```python
from build123d import *

# Parameters (mm, degrees)
SKETCH1_W           = 20.32
SKETCH1_H           = 42
BOSS_EXTRUDE1_DEPTH = 1.5748
SKETCH2_W           = 42
SKETCH2_H           = 1.5748
BOSS_EXTRUDE2_DEPTH = 62.32
SKETCH3_R           = 11.303
SKETCH3_R_2         = 1.6891
CUT_EXTRUDE1_DEPTH  = 62.32
SKETCH4_R           = 2.05
CUT_EXTRUDE2_DEPTH  = 62.32


with BuildPart() as part:
    # Sketch1 → Boss-Extrude1 (new body)
    with BuildSketch(Plane(origin=(0, 0, 0), x_dir=(0, 1, 0), z_dir=(0, 0, 1))):
        Rectangle(SKETCH1_W, SKETCH1_H)
    extrude(amount=BOSS_EXTRUDE1_DEPTH)

    # Sketch2 → Boss-Extrude2 (add)
    with BuildSketch(Plane.XY.offset(1.5748)):
        with Locations((0, 9.3726)):
            Rectangle(SKETCH2_W, SKETCH2_H)
    extrude(amount=BOSS_EXTRUDE2_DEPTH)

    # Sketch3 → Cut-Extrude1 (cut)
    with BuildSketch(Plane(origin=(0, 8.5852, 0), x_dir=(-1, 0, 0), z_dir=(0, -1, 0))):
        with Locations(Location((0, -42.8918, 0), (0, 0, 90))):
            Circle(SKETCH3_R)
        with Locations(Location((-15.5009, -58.3957, 0), (0, 0, 90))):
            Circle(SKETCH3_R_2)
        with Locations(Location((-15.5009, -27.2175, 0), (0, 0, 90))):
            Circle(SKETCH3_R_2)
        with Locations(Location((15.5009, -27.2175, 0), (0, 0, 180))):
            Circle(SKETCH3_R_2)
        with Locations(Location((15.5009, -58.3957, 0), (0, 0, 180))):
            Circle(SKETCH3_R_2)
    extrude(amount=-CUT_EXTRUDE1_DEPTH, mode=Mode.SUBTRACT)

    # Sketch4 → Cut-Extrude2 (cut)
    with BuildSketch(Plane.XY.offset(1.5748)):
        with Locations((9.035, 0)):
            Circle(SKETCH4_R)
        with Locations((-9.035, 0)):
            Circle(SKETCH4_R)
    extrude(amount=-CUT_EXTRUDE2_DEPTH, mode=Mode.SUBTRACT)


solid = part.part
```
For this review, take the finished solid that the model builds, in its own axes (mm). A direction names the side the tool comes from. Give positions to 0.01 mm unless a question says otherwise; leave off trailing zeros. Write each loop counter-clockwise with the first axis right and the second up, starting at its lowest first coordinate (ties: lowest second). Pieces come first, ordered by that corner, then holes.
Item 1: Take a section at C-C (z = 15). Give the boundary of the cut face in (x, y).
Item 2: Machinability: for faces 1 (the face through (0, -1, 1.575)), 2 (the face through (21, 9, 22)), which of the approach directions +Z, -Z, +X, -X, +Y, -Y give a long, thin tool a straight path to every point of the face, cutting with its end or side? Answer none if there is none.
Item 3: Insertion check: P1, Ø1.5, axis at x = 8.5, z = 57.5, coming from the -Y side; P2, Ø4, axis at x = 8.5, y = 3, coming from the +Z side. Each pin has a flat end and moves straight along its axis. Give the tip position at first contact, or say it passes through.
Item 4: Take a section at B-B (x = 0). Give the boundary of the cut face in (y, z).
Item 5: Wall thickness on probe 1 along Y at (x, z) = (-2.5, 19); probe 2 along Z at (x, y) = (5, -5.25): over which ranges is each line inside the solid? List them lowest first.
Item 6: Take a section at D-D (y = -7.5). Give the boundary of the cut face in (x, z).
Item 7: Take a section at A-A (y = 0). Give the boundary of the cut face in (x, z) (3 decimals), and give its area (3 significant figures).
Item 8: The part is to be moulded in two halves that separate along X. For faces 3 (the face through (-13.89, 9.36, 27.72)), 4 (the face through (-21, 9, 22)), 5 (the face through (0, 8.585, 25)), say which applies: +X half, -X half, draft (parallel to the pull), parting line (faces both ways), or undercut.
Established:
1. outline: (-21, 8.59) - (21, 8.59) - (21, 10.16) - (-21, 10.16) - close
2. face 1: +Z, +X, -X, -Y
2. face 2: +Z, -Z, +X, +Y, -Y
3. P1: stops at y = 8.59
3. P2: stops at z = 1.57
4. outline: (-10.16, 0) - (10.16, 0) - (10.16, 31.59) - (8.59, 31.59) - (8.59, 1.57) - (-10.16, 1.57) - close; (8.59, 54.19) - (10.16, 54.19) - (10.16, 63.89) - (8.59, 63.89) - close
5. probe 1: y = 8.59 to 10.16
5. probe 2: z = 0 to 1.57
6. outline: (-21, 0) - (21, 0) - (21, 1.57) - (-21, 1.57) - close
7. outline: (-21, 0) - (-11.085, 0) - (-11.085, 1.575) - (-21, 1.575) - close; (-6.985, 0) - (6.985, 0) - (6.985, 1.575) - (-6.985, 1.575) - close; (11.085, 0) - (21, 0) - (21, 1.575) - (11.085, 1.575) - close
7. area: 53.2 mm2
8. face 3: undercut
8. face 4: -X half
8. face 5: draft
